Part model, mm, in its own coordinate system. A direction names the side the tool comes from. Round coordinates to 2 decimals unless told otherwise and drop trailing zeros. Order: outer loops, then holes, each group sorted by start corner. A loop starts at its lowest first (then second) coordinate and runs counter-clockwise, first axis right, second up. Notation, with made-up numbers: (7, 56.5) - (54, 56.5) arc R35 ccw to (54, 90.5) - close; hole circle Ø8 at (41, -15). An arc over 180 degrees is marked (long way). Answer as a JSON object with one key per item and string values.
```python
from build123d import *

# Parameters (mm, degrees)
SKETCH1_W           = 50
SKETCH1_H           = 50
BOSS_EXTRUDE1_DEPTH = 5
SKETCH2_R           = 1.6
CUT_EXTRUDE1_DEPTH  = 5
SKETCH4_W           = 15
SKETCH4_H           = 15
CUT_EXTRUDE2_DEPTH  = 5
CUT_EXTRUDE3_DEPTH  = 3
FILLET2_R           = 10
FILLET3_R           = 5


with BuildPart() as part:
    # Sketch1 → Boss-Extrude1 (new body)
    with BuildSketch(Plane(origin=(0, 0, 0), x_dir=(1, 0, 0), z_dir=(0, 1, 0))):
        with Locations((-39.516129032, 6.912442396)):
            Rectangle(SKETCH1_W, SKETCH1_H)
    extrude(amount=BOSS_EXTRUDE1_DEPTH)

    # Sketch2 → Cut-Extrude1 (cut)
    with BuildSketch(Plane(origin=(0, 5, 0), x_dir=(1, 0, 0), z_dir=(0, 1, 0))):
        with Locations(Location((-57.016129032, 24.412442396, 0), (0, 0, 270))):
            Circle(SKETCH2_R)
        with Locations(Location((-22.016129032, 24.412442396, 0), (0, 0, 270))):
            Circle(SKETCH2_R)
        with Locations(Location((-57.016129032, -10.587557604, 0), (0, 0, 270))):
            Circle(SKETCH2_R)
        with Locations(Location((-22.016129032, -10.587557604, 0), (0, 0, 270))):
            Circle(SKETCH2_R)
    extrude(amount=-CUT_EXTRUDE1_DEPTH, mode=Mode.SUBTRACT)

    # Sketch4 → Cut-Extrude2 (cut)
    with BuildSketch(Plane(origin=(0, 5, 0), x_dir=(1, 0, 0), z_dir=(0, 1, 0))):
        with Locations((-39.516129032, 6.912442396)):
            Rectangle(SKETCH4_W, SKETCH4_H)
    extrude(amount=-CUT_EXTRUDE2_DEPTH, mode=Mode.SUBTRACT)

    # Sketch5 → Cut-Extrude3 (cut)
    with BuildSketch(Plane(origin=(0, 5, 0), x_dir=(1, 0, 0), z_dir=(0, 1, 0))):
        Polygon((-58.766129032, 27.44353131), (-60.516129032, 24.412442396), (-58.766129032, 21.381353483), (-55.266129032, 21.381353483), (-53.516129032, 24.412442396), (-55.266129032, 27.44353131), align=None)
        Polygon((-23.766129032, 27.44353131), (-25.516129032, 24.412442396), (-23.766129032, 21.381353483), (-20.266129032, 21.381353483), (-18.516129032, 24.412442396), (-20.266129032, 27.44353131), align=None)
        Polygon((-58.766129032, -7.55646869), (-60.516129032, -10.587557604), (-58.766129032, -13.618646517), (-55.266129032, -13.618646517), (-53.516129032, -10.587557604), (-55.266129032, -7.55646869), align=None)
        Polygon((-23.766129032, -7.55646869), (-25.516129032, -10.587557604), (-23.766129032, -13.618646517), (-20.266129032, -13.618646517), (-18.516129032, -10.587557604), (-20.266129032, -7.55646869), align=None)
    extrude(amount=-CUT_EXTRUDE3_DEPTH, mode=Mode.SUBTRACT)

    # Fillet2
    fillet2_edges = [part.edges().sort_by_distance(p)[0] for p in [
        (-64.516129032, 2.5, -31.912442396),
        (-14.516129032, 2.5, -31.912442396),
        (-14.516129032, 2.5, 18.087557604),
        (-64.516129032, 2.5, 18.087557604),
    ]]
    fillet(fillet2_edges, radius=FILLET2_R)

    # Fillet3
    fillet3_edges = [part.edges().sort_by_distance(p)[0] for p in [
        (-39.516129032, 5, -14.412442396),
        (-32.016129032, 5, -6.912442396),
        (-39.516129032, 5, 0.587557604),
        (-47.016129032, 5, -6.912442396),
    ]]
    fillet(fillet3_edges, radius=FILLET3_R - 0.0001)  # a hair under: the kernel refuses the full size


solid = part.part
```
Item 1: Tool access for faces 1 (the flat face through (-57, 4, -27.444)), 2 (the flat face through (-29, 0, -7)): list every direction of +Z, -Z, +X, -X, +Y, -Y with a clear straight run to the whole face (end or side of a thin tool).
Taken from the geometry:
{"face 1": "+Y", "face 2": "+Z, -Z, +X, -X, -Y"}
Item 2: Two-plate mould, pull along X, no slides. Class faces 3 (the flat face through (-14.516, 2, -7)), 4 (the flat face through (-23, 5, -7)), 5 (the flat face through (-23, 2, -26)): pulls with the +X half, pulls with the -X half, needs draft (parallel to the pull), parting line crosses it, or undercut.
Taken from the geometry:
{"face 3": "pulls with the +X half", "face 4": "needs draft", "face 5": "undercut"}
Item 3: Cut at C-C (z = -25). Write the cut outline in (x, y).
Taken from the geometry:
{"outline": "(-64.03, 0) - (-58.5, 0) - (-58.5, 2) - (-60.18, 2) - (-60.18, 5) - (-64.03, 5) - close; (-55.53, 0) - (-23.5, 0) - (-23.5, 2) - (-25.18, 2) - (-25.18, 5) - (-53.86, 5) - (-53.86, 2) - (-55.53, 2) - close; (-20.53, 0) - (-15, 0) - (-15, 5) - (-18.86, 5) - (-18.86, 2) - (-20.53, 2) - close"}
Item 4: Probe L1, parallel to Z at x = -20, y = 2.4; L2, parallel to Z at x = -22, y = 3.7; L3, parallel to X at y = 3.45, z = 9. List the from-to ranges inside material, lowest first. Write a range as from..to.
Taken from the geometry:
{"L1": "-30.83..-26.98, -21.84..8.02, 13.16..17.01", "L2": "-31.59..-27.44, -21.38..7.56, 13.62..17.77", "L3": "-64.47..-59.6, -54.43..-24.6, -19.43..-14.56"}
Item 5: Drop flat-ended pins along their axis: P1, Ø0.9, axis at x = -21.5, y = 3.5, coming from the -Z side; P2, Ø0.9, axis at x = -21.5, y = 3.5, coming from the +Z side; P3, Ø2.5, axis at x = -22, y = 3.5, coming from the +Z side. Give the stop position or say it passes through.
Taken from the geometry:
{"P1": "z = -31.58", "P2": "z = 17.75", "P3": "z = 18.01"}
Item 6: Cut at D-D (y = 1.05). Write the cut outline in (x, z), plus the area to 3 significant figures.
Taken from the geometry:
{"outline": "(-64.52, -21.91) arc R10 ccw to (-54.52, -31.91) - (-24.52, -31.91) arc R10 ccw to (-14.52, -21.91) - (-14.52, 8.09) arc R10 ccw to (-24.52, 18.09) - (-54.52, 18.09) arc R10 ccw to (-64.52, 8.09) - close; hole circle Ø3.2 at (-57.02, -24.41); hole circle Ø3.2 at (-57.02, 10.59); hole (-47.13, -14.52) - (-31.9, -14.52) - (-31.9, 0.7) - (-47.13, 0.7) - close; hole circle Ø3.2 at (-22.02, -24.41); hole circle Ø3.2 at (-22.02, 10.59)", "area": "2,150 mm2"}
